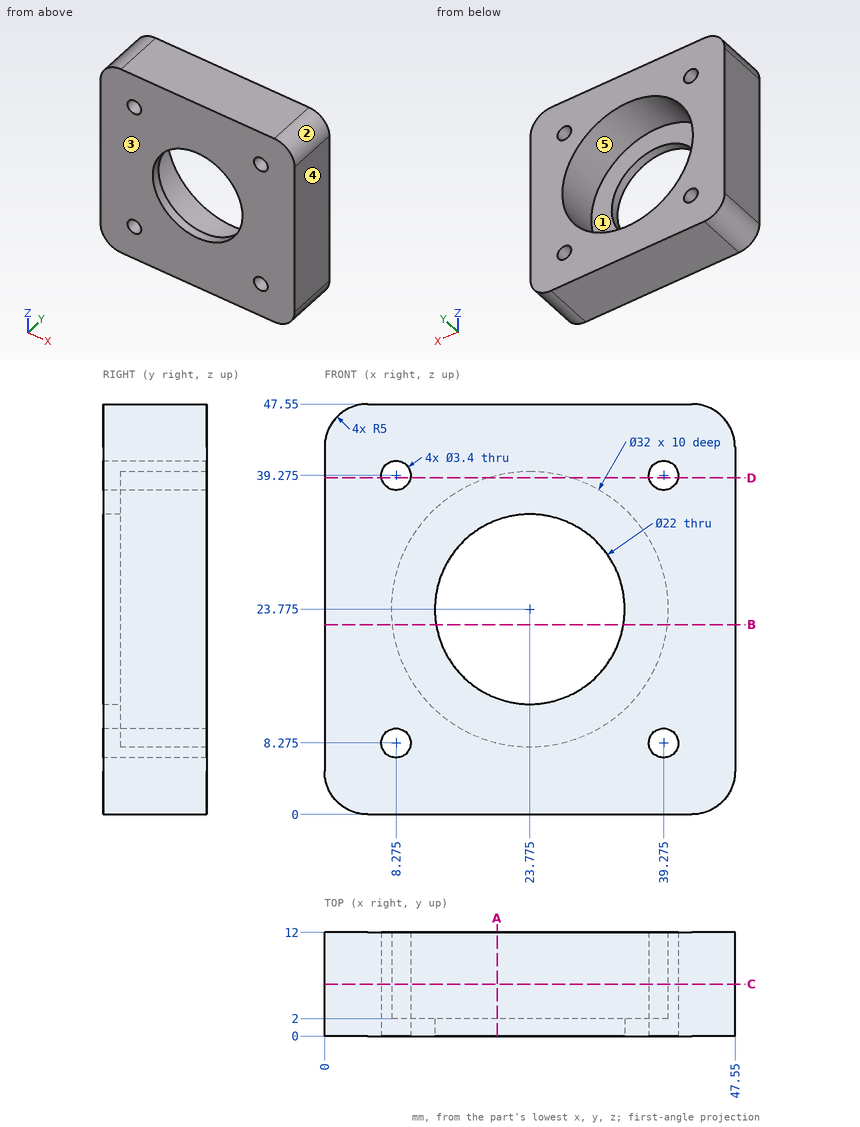
Source: three-view drawing plus pictorial views. Frame: mm from the lowest corner of the part. A direction names the side the tool comes from. Round coordinates to 2 decimals unless told otherwise and drop trailing zeros. Loops run counter-clockwise (first coordinate to the right, second up) from the corner with the lowest first, then second, coordinate; pieces in that order, holes last. Notation, with made-up numbers: (-6.5, 67.25) - (17.5, 67.25) arc R32 cw to (17.5, 93.25) - close; hole circle Ø4 at (-2, 51). An arc over 180 degrees is marked (long way). Write item = value, one per line. Start each with the question number.
Item 1: Section query A-A on x = 20. Output: boundary loops of the cut face in (y, z), plus the area to 3 significant figures.
Item 2: First-contact query: pin 1 Ø17.5 at (x, z) = (23.775, 23.775) entering from +Y; pin 2 Ø16 at (x, z) = (20, 22.5) entering from +Y. Flat tips, straight axial feed; report the tip coordinate or a pass-through.
Item 3: Mould query, pull axis X, two halves, no side actions, for the marked faces 1, 2 and 3. Classes: released by +X, released by -X, zero draft, split by the parting line, or undercut.
Item 4: Reachability of the marked faces 4 and 5 from +Z, -Z, +X, -X, +Y, -Y: full face, straight path, thin tool, end or side. Return the list, or none.
Item 5: Section query D-D on z = 39. Output: boundary loops of the cut face in (x, y), plus the area to 3 significant figures.
Item 6: Material intervals for line 1 (Z direction, x = 7, y = 2.75); line 2 (X direction, y = 9, z = 25); line 3 (Z direction, x = 37, y = 3.75), sorted ascending.
Item 7: Section query B-B on z = 22. Output: boundary loops of the cut face in (x, y), plus the area to 3 significant figures.
Item 8: Section query C-C on y = 6. Output: boundary loops of the cut face in (x, z) (3 decimals), plus the area to 3 significant figures.
Results list:
q1.outline = (0, 0) - (12, 0) - (12, 8.23) - (2, 8.23) - (2, 13.44) - (0, 13.44) - close; (0, 34.11) - (2, 34.11) - (2, 39.32) - (12, 39.32) - (12, 47.55) - (0, 47.55) - close
q1.area = 218 mm²
q2.pin_1 = through
q2.pin_2 = 2
q3.face_1 = undercut
q3.face_2 = released by +X
q3.face_3 = zero draft
q4.face_4 = +Z, -Z, +X, +Y, -Y
q4.face_5 = +Y
q5.outline = (0, 0) - (6.6, 0) - (6.6, 12) - (0, 12) - close; (9.95, 0) - (37.6, 0) - (37.6, 12) - (28.69, 12) - (28.69, 2) - (18.86, 2) - (18.86, 12) - (9.95, 12) - close; (40.95, 0) - (47.55, 0) - (47.55, 12) - (40.95, 12) - close
q5.area = 392 mm²
q6.line_1 = 0 to 7.15, 9.4 to 38.15, 40.4 to 47.55
q6.line_2 = 0 to 7.82, 39.73 to 47.55
q6.line_3 = 0 to 14.77, 32.78 to 47.55
q7.outline = (0, 0) - (12.92, 0) - (12.92, 2) - (7.87, 2) - (7.87, 12) - (0, 12) - close; (34.63, 0) - (47.55, 0) - (47.55, 12) - (39.68, 12) - (39.68, 2) - (34.63, 2) - close
q7.area = 209 mm²
q8.outline = (0, 5) arc R5 ccw to (5, 0) - (42.55, 0) arc R5 ccw to (47.55, 5) - (47.55, 42.55) arc R5 ccw to (42.55, 47.55) - (5, 47.55) arc R5 ccw to (0, 42.55) - close; hole circle Ø3.4 at (8.275, 8.275); hole circle Ø3.4 at (8.275, 39.275); hole circle Ø32 at (23.775, 23.775); hole circle Ø3.4 at (39.275, 8.275); hole circle Ø3.4 at (39.275, 39.275)
q8.area = 1,400 mm²
